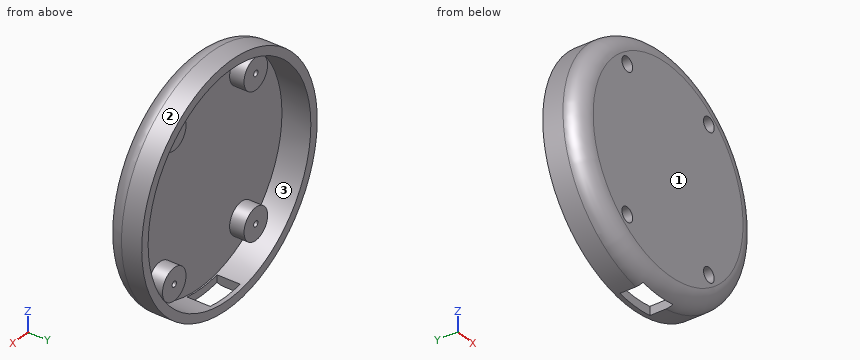
from build123d import *

# Parameters (mm, degrees)
SKETCH1_R           = 41
SKETCH1_R_2         = 2.5
BOSS_EXTRUDE1_DEPTH = 3
SKETCH3_R           = 41
SKETCH3_R_2         = 38
BOSS_EXTRUDE2_DEPTH = 10
SKETCH3_3_R         = 5.5
SKETCH3_3_R_2       = 2.5
BOSS_EXTRUDE3_DEPTH = 3
SKETCH4_R           = 5.5
SKETCH4_R_2         = 1
BOSS_EXTRUDE4_DEPTH = 2
FILLET1_R           = 6
SKETCH6_W           = 14
SKETCH6_H           = 8
CUT_EXTRUDE1_DEPTH  = 60.422218067


with BuildPart() as part:
    # Sketch1 → Boss-Extrude1 (new body)
    with BuildSketch(Plane(origin=(0, 0, 0), x_dir=(1, 0, 0), z_dir=(0, 1, 0))):
        with Locations(Location((0, 0, 0), (0, 0, 270))):
            Circle(SKETCH1_R)
        with Locations(Location((-19.05, 25, 0), (0, 0, 270))):
            Circle(SKETCH1_R_2, mode=Mode.SUBTRACT)
        with Locations(Location((19.05, 25, 0), (0, 0, 270))):
            Circle(SKETCH1_R_2, mode=Mode.SUBTRACT)
        with Locations(Location((19.05, -25, 0), (0, 0, 270))):
            Circle(SKETCH1_R_2, mode=Mode.SUBTRACT)
        with Locations(Location((-19.05, -25, 0), (0, 0, 270))):
            Circle(SKETCH1_R_2, mode=Mode.SUBTRACT)
    extrude(amount=BOSS_EXTRUDE1_DEPTH)

    # Sketch3 → Boss-Extrude2 (add)
    with BuildSketch(Plane(origin=(0, 3, 0), x_dir=(1, 0, 0), z_dir=(0, 1, 0))):
        with Locations(Location((0, 0, 0), (0, 0, 270))):
            Circle(SKETCH3_R)
        with Locations(Location((0, 0, 0), (0, 0, 270))):
            Circle(SKETCH3_R_2, mode=Mode.SUBTRACT)
    extrude(amount=BOSS_EXTRUDE2_DEPTH)

    # Sketch3_3 → Boss-Extrude3 (add)
    # profile 1 of 4: a face of its own
    with BuildSketch(Plane(origin=(0, 3, 0), x_dir=(1, 0, 0), z_dir=(0, 1, 0))):
        with Locations(Location((-19.05, 25, 0), (0, 0, 270))):
            Circle(SKETCH3_3_R)
        with Locations(Location((-19.05, 25, 0), (0, 0, 270))):
            Circle(SKETCH3_3_R_2, mode=Mode.SUBTRACT)
    # profile 2 of 4: a face of its own
    with BuildSketch(Plane(origin=(0, 3, 0), x_dir=(1, 0, 0), z_dir=(0, 1, 0))):
        with Locations(Location((19.05, 25, 0), (0, 0, 270))):
            Circle(SKETCH3_3_R)
        with Locations(Location((19.05, 25, 0), (0, 0, 270))):
            Circle(SKETCH3_3_R_2, mode=Mode.SUBTRACT)
    # profile 3 of 4: a face of its own
    with BuildSketch(Plane(origin=(0, 3, 0), x_dir=(1, 0, 0), z_dir=(0, 1, 0))):
        with Locations(Location((-19.05, -25, 0), (0, 0, 270))):
            Circle(SKETCH3_3_R)
        with Locations(Location((-19.05, -25, 0), (0, 0, 270))):
            Circle(SKETCH3_3_R_2, mode=Mode.SUBTRACT)
    # profile 4 of 4: a face of its own
    with BuildSketch(Plane(origin=(0, 3, 0), x_dir=(1, 0, 0), z_dir=(0, 1, 0))):
        with Locations(Location((19.05, -25, 0), (0, 0, 270))):
            Circle(SKETCH3_3_R)
        with Locations(Location((19.05, -25, 0), (0, 0, 270))):
            Circle(SKETCH3_3_R_2, mode=Mode.SUBTRACT)
    extrude(amount=BOSS_EXTRUDE3_DEPTH)

    # Sketch4 → Boss-Extrude4 (add)
    # profile 1 of 4: a face of its own
    with BuildSketch(Plane(origin=(0, 6, 0), x_dir=(1, 0, 0), z_dir=(0, 1, 0))):
        with Locations(Location((-19.05, 25, 0), (0, 0, 270))):
            Circle(SKETCH4_R)
        with Locations(Location((-19.05, 25, 0), (0, 0, 270))):
            Circle(SKETCH4_R_2, mode=Mode.SUBTRACT)
    # profile 2 of 4: a face of its own
    with BuildSketch(Plane(origin=(0, 6, 0), x_dir=(1, 0, 0), z_dir=(0, 1, 0))):
        with Locations(Location((19.05, 25, 0), (0, 0, 270))):
            Circle(SKETCH4_R)
        with Locations(Location((19.05, 25, 0), (0, 0, 270))):
            Circle(SKETCH4_R_2, mode=Mode.SUBTRACT)
    # profile 3 of 4: a face of its own
    with BuildSketch(Plane(origin=(0, 6, 0), x_dir=(1, 0, 0), z_dir=(0, 1, 0))):
        with Locations(Location((19.05, -25, 0), (0, 0, 270))):
            Circle(SKETCH4_R)
        with Locations(Location((19.05, -25, 0), (0, 0, 270))):
            Circle(SKETCH4_R_2, mode=Mode.SUBTRACT)
    # profile 4 of 4: a face of its own
    with BuildSketch(Plane(origin=(0, 6, 0), x_dir=(1, 0, 0), z_dir=(0, 1, 0))):
        with Locations(Location((-19.05, -25, 0), (0, 0, 270))):
            Circle(SKETCH4_R)
        with Locations(Location((-19.05, -25, 0), (0, 0, 270))):
            Circle(SKETCH4_R_2, mode=Mode.SUBTRACT)
    extrude(amount=BOSS_EXTRUDE4_DEPTH)

    # Fillet1
    fillet1_edges = [part.edges().sort_by_distance(p)[0] for p in [
        (0, 0, -41),
    ]]
    fillet(fillet1_edges, radius=FILLET1_R)

    # Sketch6 → Cut-Extrude1 (cut, through all)
    with BuildSketch(Plane.XY):
        with Locations((0, 7.5)):
            Rectangle(SKETCH6_W, SKETCH6_H)
    extrude(amount=-CUT_EXTRUDE1_DEPTH, mode=Mode.SUBTRACT)


solid = part.part
Source: CAD feature listing. Evaluate the final solid. Frame: model axes, mm. Face numbers are marked on the shaded views. Give positions to 0.01 mm unless a question says otherwise; leave off trailing zeros. Order: outer loops, then holes, each group sorted by start corner. A loop starts at its lowest first (then second) coordinate and runs counter-clockwise, first axis right, second up. Notation, with made-up numbers: (55.5, 40) -> (70.5, 40) arc R32 cw to (70.5, 73) -> close; hole circle Ø2 at (46, 87). An arc over 180 degrees is marked (long way). Use a Markdown table: item, result.
1) Mould query, pull axis X, two halves, no side actions, for the marked faces 1, 2 and 3. Classes: +X half, -X half, draft (parallel to the pull), parting line (faces both ways), or undercut.
Answer list:
| item | result |
|---|---|
| face 1 | draft |
| face 2 | parting line |
| face 3 | undercut |
2) Section query C-C, the plane z = -25. Count the separate pieces of the cut face and the enclosed holes in it, then the cut area to 3 significant figures.
Answer list:
| item | result |
|---|---|
| separate pieces | 3 |
| enclosed holes | 0 |
| area | 295 mm² |
3) Ray query, line 1 along Z through (x, y) = (-15, 6.25); line 2 along X through (y, z) = (11.25, 0); line 3 along X through (y, z) = (5.5, -28). Return the intervals inside material, ascending. Write a range as [from, to].
Answer list:
| item | result |
|---|---|
| line 1 | [-38.16, -34.91], [-28.72, -21.28], [21.28, 28.72], [34.91, 38.16] |
| line 2 | [-41, -38], [38, 41] |
| line 3 | [-29.92, -25.69], [-23.66, -14.44], [14.44, 23.66], [25.69, 29.92] |
4) Section query B-B, the plane z = 0. Return the cut outline in (x, y).
Answer list:
| item | result |
|---|---|
| outline | (-41, 6) arc R6 ccw to (-35, 0) -> (35, 0) arc R6 ccw to (41, 6) -> (41, 13) -> (38, 13) -> (38, 3) -> (-38, 3) -> (-38, 13) -> (-41, 13) -> close |
5) Section query A-A, the plane x = 0. Return the cut outline in (y, z).
Answer list:
| item | result |
|---|---|
| outline | (0, -35) arc R6 ccw to (3.5, -40.45) -> (3.5, -38) -> (3, -38) -> (3, 38) -> (13, 38) -> (13, 41) -> (6, 41) arc R6 ccw to (0, 35) -> close; (11.5, -41) -> (13, -41) -> (13, -38) -> (11.5, -38) -> close |
6) Contact query for flat-ended pins moving along their axis: P1, Ø12, axis at x = 20.5, z = 24.5, coming from the +Y side; P2, Ø4.5, axis at x = 19.05, z = -25, coming from the -Y side; P3, Ø1.5, axis at y = 5, z = -26.5, coming from the -X side; P4, Ø2, axis at x = -10, z = -11.5, coming from the -Y side. Output: stop coordinate, or through.
Answer list:
| item | result |
|---|---|
| P1 | y = 8 |
| P2 | y = 6 |
| P3 | x = -31.82 |
| P4 | y = 0 |
